The model under review builds one solid part; all positions refer to its coordinate system, in mm. A direction names the side the tool comes from. Give positions to 0.01 mm unless a question says otherwise; leave off trailing zeros. Order: outer loops, then holes, each group sorted by start corner. A loop starts at its lowest first (then second) coordinate and runs counter-clockwise, first axis right, second up. Notation, with made-up numbers: (66, 65) - (85, 65) arc R23 ccw to (85, 73) - close; hole circle Ø11 at (-15.75, 45.5). An arc over 180 degrees is marked (long way). Use a Markdown table: item, result. Add a question column.
```python
from build123d import *

# Parameters (mm, degrees)
SKETCH_1_W          = 105
SKETCH_1_H          = 50
EXTRUDE_1_DEPTH     = 2
FILLET_1_R          = 11
SKETCH_3_R          = 2.15
CUT_EXTRUDE_1_DEPTH = 1
CUT_EXTRUDE_2_REACH = 60.157
SKETCH_4_R          = 1.15
CUT_EXTRUDE_3_REACH = 60.183
SKETCH_5_W          = 9.2
SKETCH_5_H          = 3.5
SKETCH_6_W          = 34.3
SKETCH_6_H          = 24.3
SKETCH_6_W_2        = 30.3
SKETCH_6_H_2        = 20.3
EXTRUDE_1_2_DEPTH   = 4
SKETCH_7_R          = 1.25
CUT_EXTRUDE_4_DEPTH = 2
SKETCH_8_W          = 2
SKETCH_8_H          = 15
CUT_EXTRUDE_5_DEPTH = 4


with BuildPart() as part:
    # 草图1 → Extrude 1 (new body)
    with BuildSketch(Plane.XY):
        Rectangle(SKETCH_1_W, SKETCH_1_H)
    extrude(amount=EXTRUDE_1_DEPTH)

    # 圆角1
    fillet_1_edges = [part.edges().sort_by_distance(p)[0] for p in [
        (52.5, -25, 1),
        (-52.5, -25, 1),
        (-52.5, 25, 1),
        (52.5, 25, 1),
    ]]
    fillet(fillet_1_edges, radius=FILLET_1_R)

    # 草图3 → 切除-拉伸1 (cut)
    with BuildSketch(Plane(origin=(0, 0, 0), x_dir=(-1, 0, 0), z_dir=(0, 0, -1))):
        with Locations((47.88083152, -20)):
            Circle(SKETCH_3_R)
        with Locations((47.88083152, 20)):
            Circle(SKETCH_3_R)
        with Locations((-47.88083152, 20)):
            Circle(SKETCH_3_R)
        with Locations((-47.88083152, -20)):
            Circle(SKETCH_3_R)
    extrude(amount=-CUT_EXTRUDE_1_DEPTH, mode=Mode.SUBTRACT)

    # 草图4 → 切除-拉伸2 (cut, up to next)
    with BuildSketch(Plane(origin=(0, 0, 1), x_dir=(-1, 0, 0), z_dir=(0, 0, -1)), mode=Mode.PRIVATE) as cut_extrude_2_sk1:
        with Locations((47.88083152, -20)):
            Circle(SKETCH_4_R)
    cut_extrude_2_tool1 = extrude(cut_extrude_2_sk1.sketch, amount=-CUT_EXTRUDE_2_REACH, mode=Mode.PRIVATE) & part.part
    # 草图4 → 切除-拉伸2 (cut, up to next)
    with BuildSketch(Plane(origin=(0, 0, 1), x_dir=(-1, 0, 0), z_dir=(0, 0, -1)), mode=Mode.PRIVATE) as cut_extrude_2_sk2:
        with Locations((-47.88083152, -20)):
            Circle(SKETCH_4_R)
    cut_extrude_2_tool2 = extrude(cut_extrude_2_sk2.sketch, amount=-CUT_EXTRUDE_2_REACH, mode=Mode.PRIVATE) & part.part
    # 草图4 → 切除-拉伸2 (cut, up to next)
    with BuildSketch(Plane(origin=(0, 0, 1), x_dir=(-1, 0, 0), z_dir=(0, 0, -1)), mode=Mode.PRIVATE) as cut_extrude_2_sk3:
        with Locations((47.88083152, 20)):
            Circle(SKETCH_4_R)
    cut_extrude_2_tool3 = extrude(cut_extrude_2_sk3.sketch, amount=-CUT_EXTRUDE_2_REACH, mode=Mode.PRIVATE) & part.part
    # 草图4 → 切除-拉伸2 (cut, up to next)
    with BuildSketch(Plane(origin=(0, 0, 1), x_dir=(-1, 0, 0), z_dir=(0, 0, -1)), mode=Mode.PRIVATE) as cut_extrude_2_sk4:
        with Locations((-47.88083152, 20)):
            Circle(SKETCH_4_R)
    cut_extrude_2_tool4 = extrude(cut_extrude_2_sk4.sketch, amount=-CUT_EXTRUDE_2_REACH, mode=Mode.PRIVATE) & part.part
    add(cut_extrude_2_tool1.solids().sort_by_distance((-47.880832, -20, 1))[0], mode=Mode.SUBTRACT)
    add(cut_extrude_2_tool2.solids().sort_by_distance((47.880832, -20, 1))[0], mode=Mode.SUBTRACT)
    add(cut_extrude_2_tool3.solids().sort_by_distance((-47.880832, 20, 1))[0], mode=Mode.SUBTRACT)
    add(cut_extrude_2_tool4.solids().sort_by_distance((47.880832, 20, 1))[0], mode=Mode.SUBTRACT)

    # 草图5 → 切除-拉伸3 (cut, up to next)
    with BuildSketch(Plane(origin=(0, 0, 0), x_dir=(-1, 0, 0), z_dir=(0, 0, -1)), mode=Mode.PRIVATE) as cut_extrude_3_sk1:
        with Locations((9.5, 10.75)):
            Rectangle(SKETCH_5_W, SKETCH_5_H)
    cut_extrude_3_tool1 = extrude(cut_extrude_3_sk1.sketch, amount=-CUT_EXTRUDE_3_REACH, mode=Mode.PRIVATE) & part.part
    add(cut_extrude_3_tool1.solids().sort_by_distance((-9.5, 10.75, 0))[0], mode=Mode.SUBTRACT)

    # 草图6 → Extrude 1 2 (add)
    with BuildSketch(Plane.XY.offset(2)):
        with Locations((-18.85, -5.15)):
            Rectangle(SKETCH_6_W, SKETCH_6_H)
        with Locations((-18.85, -5.15)):
            Rectangle(SKETCH_6_W_2, SKETCH_6_H_2, mode=Mode.SUBTRACT)
    extrude(amount=EXTRUDE_1_2_DEPTH)

    # 草图7 → 切除-拉伸4 (cut)
    with BuildSketch(Plane.XY.offset(2)):
        with Locations(Location((-32.75, 3.75, 0), (0, 0, 180))):
            Circle(SKETCH_7_R)
        with Locations(Location((-29.67, 3.75, 0), (0, 0, 90))):
            Circle(SKETCH_7_R)
        with Locations(Location((-26.59, 3.75, 0), (0, 0, 90))):
            Circle(SKETCH_7_R)
        with Locations(Location((-23.51, 3.75, 0), (0, 0, 90))):
            Circle(SKETCH_7_R)
        with Locations(Location((-20.43, 3.75, 0), (0, 0, 90))):
            Circle(SKETCH_7_R)
        with Locations(Location((-17.35, 3.75, 0), (0, 0, 90))):
            Circle(SKETCH_7_R)
        with Locations(Location((-14.27, 3.75, 0), (0, 0, 90))):
            Circle(SKETCH_7_R)
        with Locations(Location((-11.19, 3.75, 0), (0, 0, 90))):
            Circle(SKETCH_7_R)
        with Locations(Location((-8.11, 3.75, 0), (0, 0, 90))):
            Circle(SKETCH_7_R)
        with Locations(Location((-5.03, 3.75, 0), (0, 0, 90))):
            Circle(SKETCH_7_R)
        with Locations((-29.67, 0.77)):
            Circle(SKETCH_7_R)
        with Locations((-26.59, 0.77)):
            Circle(SKETCH_7_R)
        with Locations((-23.51, 0.77)):
            Circle(SKETCH_7_R)
        with Locations((-20.43, 0.77)):
            Circle(SKETCH_7_R)
        with Locations((-17.35, 0.77)):
            Circle(SKETCH_7_R)
        with Locations((-14.27, 0.77)):
            Circle(SKETCH_7_R)
        with Locations((-11.19, 0.77)):
            Circle(SKETCH_7_R)
        with Locations((-8.11, 0.77)):
            Circle(SKETCH_7_R)
        with Locations((-5.03, 0.77)):
            Circle(SKETCH_7_R)
        with Locations((-29.67, -2.21)):
            Circle(SKETCH_7_R)
        with Locations((-26.59, -2.21)):
            Circle(SKETCH_7_R)
        with Locations((-23.51, -2.21)):
            Circle(SKETCH_7_R)
        with Locations((-20.43, -2.21)):
            Circle(SKETCH_7_R)
        with Locations((-17.35, -2.21)):
            Circle(SKETCH_7_R)
        with Locations((-14.27, -2.21)):
            Circle(SKETCH_7_R)
        with Locations((-11.19, -2.21)):
            Circle(SKETCH_7_R)
        with Locations((-8.11, -2.21)):
            Circle(SKETCH_7_R)
        with Locations((-5.03, -2.21)):
            Circle(SKETCH_7_R)
        with Locations((-29.67, -5.19)):
            Circle(SKETCH_7_R)
        with Locations((-26.59, -5.19)):
            Circle(SKETCH_7_R)
        with Locations((-23.51, -5.19)):
            Circle(SKETCH_7_R)
        with Locations((-20.43, -5.19)):
            Circle(SKETCH_7_R)
        with Locations((-17.35, -5.19)):
            Circle(SKETCH_7_R)
        with Locations((-14.27, -5.19)):
            Circle(SKETCH_7_R)
        with Locations((-11.19, -5.19)):
            Circle(SKETCH_7_R)
        with Locations((-8.11, -5.19)):
            Circle(SKETCH_7_R)
        with Locations((-5.03, -5.19)):
            Circle(SKETCH_7_R)
        with Locations((-29.67, -8.17)):
            Circle(SKETCH_7_R)
        with Locations((-26.59, -8.17)):
            Circle(SKETCH_7_R)
        with Locations((-23.51, -8.17)):
            Circle(SKETCH_7_R)
        with Locations((-20.43, -8.17)):
            Circle(SKETCH_7_R)
        with Locations((-17.35, -8.17)):
            Circle(SKETCH_7_R)
        with Locations((-14.27, -8.17)):
            Circle(SKETCH_7_R)
        with Locations((-11.19, -8.17)):
            Circle(SKETCH_7_R)
        with Locations((-8.11, -8.17)):
            Circle(SKETCH_7_R)
        with Locations((-5.03, -8.17)):
            Circle(SKETCH_7_R)
        with Locations((-29.67, -11.15)):
            Circle(SKETCH_7_R)
        with Locations((-26.59, -11.15)):
            Circle(SKETCH_7_R)
        with Locations((-23.51, -11.15)):
            Circle(SKETCH_7_R)
        with Locations((-20.43, -11.15)):
            Circle(SKETCH_7_R)
        with Locations((-17.35, -11.15)):
            Circle(SKETCH_7_R)
        with Locations((-14.27, -11.15)):
            Circle(SKETCH_7_R)
        with Locations((-11.19, -11.15)):
            Circle(SKETCH_7_R)
        with Locations((-8.11, -11.15)):
            Circle(SKETCH_7_R)
        with Locations((-5.03, -11.15)):
            Circle(SKETCH_7_R)
        with Locations(Location((-29.67, -14.13, 0), (0, 0, 290.609692938))):
            Circle(SKETCH_7_R)
        with Locations(Location((-26.59, -14.13, 0), (0, 0, 290.609692938))):
            Circle(SKETCH_7_R)
        with Locations(Location((-23.51, -14.13, 0), (0, 0, 290.609692938))):
            Circle(SKETCH_7_R)
        with Locations(Location((-20.43, -14.13, 0), (0, 0, 290.609692938))):
            Circle(SKETCH_7_R)
        with Locations(Location((-17.35, -14.13, 0), (0, 0, 290.609692938))):
            Circle(SKETCH_7_R)
        with Locations(Location((-14.27, -14.13, 0), (0, 0, 290.609692938))):
            Circle(SKETCH_7_R)
        with Locations(Location((-11.19, -14.13, 0), (0, 0, 290.609692938))):
            Circle(SKETCH_7_R)
        with Locations(Location((-8.11, -14.13, 0), (0, 0, 290.609692938))):
            Circle(SKETCH_7_R)
        with Locations(Location((-5.03, -14.13, 0), (0, 0, 290.609692938))):
            Circle(SKETCH_7_R)
        with Locations(Location((-32.75, 0.77, 0), (0, 0, 180))):
            Circle(SKETCH_7_R)
        with Locations(Location((-32.75, -2.21, 0), (0, 0, 180))):
            Circle(SKETCH_7_R)
        with Locations(Location((-32.75, -5.19, 0), (0, 0, 180))):
            Circle(SKETCH_7_R)
        with Locations(Location((-32.75, -8.17, 0), (0, 0, 180))):
            Circle(SKETCH_7_R)
        with Locations(Location((-32.75, -11.15, 0), (0, 0, 180))):
            Circle(SKETCH_7_R)
        with Locations(Location((-32.75, -14.13, 0), (0, 0, 180))):
            Circle(SKETCH_7_R)
    extrude(amount=-CUT_EXTRUDE_4_DEPTH, mode=Mode.SUBTRACT)

    # 草图8 → 切除-拉伸5 (cut)
    with BuildSketch(Plane.XY.offset(6)):
        with Locations((-35, -5.24)):
            Rectangle(SKETCH_8_W, SKETCH_8_H)
    extrude(amount=-CUT_EXTRUDE_5_DEPTH, mode=Mode.SUBTRACT)


solid = part.part
```
Q1. Clearance check with flat-ended pins moving along their axes: P1, Ø3, axis at x = -11.19, y = -5.19, coming from the +Z side; P2, Ø2, axis at x = -23.51, y = -5.19, coming from the +Z side; P3, Ø2, axis at x = -15, z = 3.5, coming from the -Y side. State where each tip first meets the part, or that it passes through.
Q2. Wall thickness on probe 1 along X at (y, z) = (11, 0.65); probe 2 along Y at (x, z) = (-7, 3.5); probe 3 along Y at (x, z) = (-12.5, 1.3): over which ranges is each line inside the solid? List them lowest first.
Q3. Draft analysis for pull direction X (two halves, no side actions). For faces 4 (the cylindrical face through (-49.363, 21.692, 1.236)), 5 (the flat face through (-1.7, -5, 4)), 6 (the cylindrical face through (-21.68, -5.14, 1.01)), state which applies: pulls with the +X half, pulls with the -X half, needs draft (parallel to the pull), parting line crosses it, or undercut.
Q4. We need section B-B (y = -11.15). Count the separate pieces of the cut face and the enclosed holes in it, plus the area to 3 significant figures.
Q5. We need section D-D (y = -20). Write out the cut boundary in (x, z), plus the area to 3 significant figures.
Q6. We need section A-A (z = 3.7). Write out the cut boundary in (x, y).
Q7. Machinability: for faces 1 (the flat face through (-19, 5, 4)), 2 (the flat face through (47, 19, 1)), 3 (the cylindrical face through (-13.693, -12.259, 1.014)), which of the approach directions +Z, -Z, +X, -X, +Y, -Y give a long, thin tool a straight path to every point of the face, cutting with its end or side? Answer none if there is none.
Q8. We need section C-C (y = 6). Write out the cut boundary in (x, z), plus the area to 3 significant figures.
Here are the results:
| question | item | result |
|---|---|---|
| 1 | P1 | z = 2 |
| 1 | P2 | through |
| 1 | P3 | y = -17.3 |
| 2 | probe 1 | -52.5 to -14.1, -4.9 to 52.5 |
| 2 | probe 2 | -17.3 to -15.3, 5 to 7 |
| 2 | probe 3 | -25 to 9, 12.5 to 25 |
| 3 | face 4 | pulls with the -X half |
| 3 | face 5 | pulls with the +X half |
| 3 | face 6 | undercut |
| 4 | separate pieces | 11 |
| 4 | enclosed holes | 0 |
| 4 | area | 168 mm2 |
| 5 | outline | (-50.72, 0) - (-50.03, 0) - (-50.03, 1) - (-49.03, 1) - (-49.03, 2) - (-50.72, 2) - close; (-46.73, 1) - (-45.73, 1) - (-45.73, 0) - (45.73, 0) - (45.73, 1) - (46.73, 1) - (46.73, 2) - (-46.73, 2) - close; (49.03, 1) - (50.03, 1) - (50.03, 0) - (50.72, 0) - (50.72, 2) - (49.03, 2) - close |
| 5 | area | 190 mm2 |
| 6 | outline | (-36, -17.3) - (-1.7, -17.3) - (-1.7, 7) - (-36, 7) - (-36, 2.26) - (-34, 2.26) - (-34, 5) - (-3.7, 5) - (-3.7, -15.3) - (-34, -15.3) - (-34, -12.74) - (-36, -12.74) - close |
| 7 | face 1 | +Z |
| 7 | face 2 | -Z |
| 7 | face 3 | +Z, -Z |
| 8 | outline | (-52.5, 0) - (52.5, 0) - (52.5, 2) - (-1.7, 2) - (-1.7, 6) - (-36, 6) - (-36, 2) - (-52.5, 2) - close |
| 8 | area | 347 mm2 |
